Model file for the job. Use its own axes, mm. Face numbers are marked on the shaded views. Round coordinates to 2 decimals unless told otherwise and drop trailing zeros. Write each loop counter-clockwise with the first axis right and the second up, starting at its lowest first coordinate (ties: lowest second). Pieces come first, ordered by that corner, then holes.
```python
from build123d import *

# Parameters (mm, degrees)
SKETCH1_W           = 25
SKETCH1_H           = 5
BOSS_EXTRUDE1_DEPTH = 5
SKETCH2_R           = 1.25
CUT_EXTRUDE1_DEPTH  = 14.693063938
FILLET1_R           = 2.5


with BuildPart() as part:
    # Sketch1 → Boss-Extrude1 (new body)
    with BuildSketch(Plane(origin=(0, 0, 0), x_dir=(1, 0, 0), z_dir=(0, 1, 0))):
        Rectangle(SKETCH1_W, SKETCH1_H)
    extrude(amount=BOSS_EXTRUDE1_DEPTH)

    # Sketch2 → Cut-Extrude1 (cut, through all)
    with BuildSketch(Plane(origin=(0, 5, 0), x_dir=(1, 0, 0), z_dir=(0, 1, 0))):
        with Locations(Location((-10, 0, 0), (0, 0, 270))):
            Circle(SKETCH2_R)
        with Locations(Location((10, 0, 0), (0, 0, 270))):
            Circle(SKETCH2_R)
    extrude(amount=-CUT_EXTRUDE1_DEPTH, mode=Mode.SUBTRACT)

    # Fillet1
    fillet1_edges = [part.edges().sort_by_distance(p)[0] for p in [
        (12.5, 2.5, 2.5),
        (12.5, 2.5, -2.5),
        (-12.5, 2.5, 2.5),
        (-12.5, 2.5, -2.5),
    ]]
    fillet(fillet1_edges, radius=FILLET1_R - 0.0001)  # a hair under: the kernel refuses the full size


solid = part.part
```
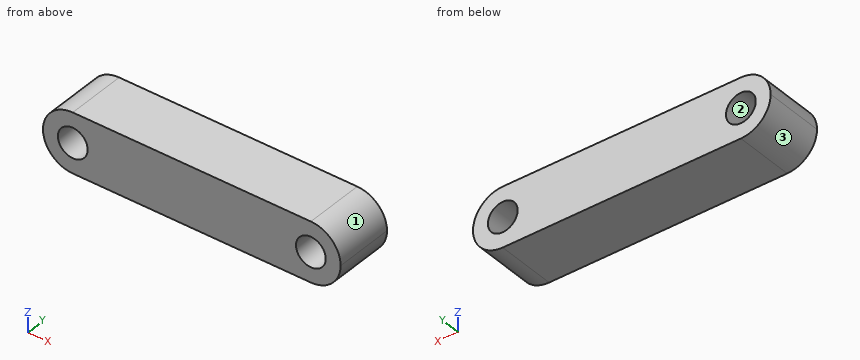
1) Pull direction Z, two halves, no side cores. Call the marked faces 1, 2 and 3: released by +Z, released by -Z, zero draft, split by the parting line, or undercut.
2) Cut at A-A on y = 2.7. Give the number of separate pieces and of enclosed holes in the cut face, and give its area (3 significant figures).
3) Cut at B-B on z = -0.3. List the corners of the cut face in (x, y).
4) Flat gauge pins, fed straight in: pin 1 Ø1 at (x, z) = (-6, 0) entering from -Y; pin 2 Ø1.5 at (y, z) = (2.5, -1.5) entering from -X. Where does each tip first touch, or does it go through?
5) Wall check: probe 1 along X at (y, z) = (1.3, 0); probe 2 along X at (y, z) = (2.3, -0.65); probe 3 along Z at (x, y) = (-10.5, 2.6). Give the ranges that are in metal, low to high.
6) Cut at C-C on z = 0.85. List the corners of the cut face in (x, y), and give its area (3 significant figures).
Result sheet:
1. face 1: released by +Z
1. face 2: undercut
1. face 3: released by -Z
2. separate pieces: 1
2. enclosed holes: 2
2. area: 110 mm2
3. outline: (-12.48, 0) - (-11.21, 0) - (-11.21, 5) - (-12.48, 5) - close; (-8.79, 0) - (8.79, 0) - (8.79, 5) - (-8.79, 5) - close; (11.21, 0) - (12.48, 0) - (12.48, 5) - (11.21, 5) - close
4. pin 1: stops at y = 0
4. pin 2: stops at x = -12.38
5. probe 1: x = -12.5 to -11.25, -8.75 to 8.75, 11.25 to 12.5
5. probe 2: x = -12.41 to -11.07, -8.93 to 8.93, 11.07 to 12.41
5. probe 3: z = -2.45 to -1.15, 1.15 to 2.45
6. outline: (-12.35, 0) - (-10.92, 0) - (-10.92, 5) - (-12.35, 5) - close; (-9.08, 0) - (9.08, 0) - (9.08, 5) - (-9.08, 5) - close; (10.92, 0) - (12.35, 0) - (12.35, 5) - (10.92, 5) - close
6. area: 105 mm2
